Geometry: final body of the model. Coordinates: model frame, mm. Give positions to 0.01 mm unless a question says otherwise; leave off trailing zeros. Order: outer loops, then holes, each group sorted by start corner. A loop starts at its lowest first (then second) coordinate and runs counter-clockwise, first axis right, second up. Notation, with made-up numbers: (85.25, 7) - (140.25, 7) arc R35 cw to (140.25, 45) - close; hole circle Ø2 at (57.25, 52.5). An arc over 180 degrees is marked (long way). Use one line per item in the form item = value.
Autodesk Inventor part; units mm, degrees
ref_plane "YZ Plane" through (0, 0, 0) normal (1, 0, 0) x (0, 1, 0)
ref_plane "XZ Plane" through (0, 0, 0) normal (0, 1, 0) x (-1, 0, 0)
ref_plane "XY Plane" through (0, 0, 0) normal (0, 0, 1) x (1, 0, 0)
sketch "Sketch1" plane through (0, 0, 0) normal (0, 1, 0) x (-1, 0, 0)
  line L0 (11.02, 0) -> (0, 0)
  line L1 (-5, -122) -> (0, -122)
  line L2 (11.02, 0) -> (11.02, -122)
  line L3 (11.02, 0) -> (133.02, 0) construction
  line L4 (11.02, -122) -> (0, -122)
  line L5 (0, -126) -> (0, -122)
  line L6 (-5, -126) -> (-5, -122)
  line L7 (0, -126) -> (-5, -126)
  line L8 (-35, -122) -> (-30, -122)
  line L9 (-30, 0) -> (-35, 0)
  line L10 (0, -122) -> (-35, -122)
  line L11 (-35, -122) -> (-35, 0)
  line L12 (0, 0) -> (-35, 0)
  line L13 (-35, 0) -> (-35, 4)
  line L14 (-35, 4) -> (-30, 4)
  line L15 (-30, 0) -> (-30, 4)
  line L16 (-20, 0) -> (-20, 4)
  line L17 (-25, 4) -> (-20, 4)
  line L18 (-25, 0) -> (-25, 4)
  line L19 (-15, 0) -> (-15, 4)
  line L20 (-15, 4) -> (-10, 4)
  line L21 (-10, 0) -> (-10, 4)
  line L22 (0, 0) -> (0, 4)
  line L23 (-5, 4) -> (0, 4)
  line L24 (-5, 0) -> (-5, 4)
  line L25 (0, -126) -> (-5, -126)
  line L26 (-10, -126) -> (-10, -122)
  line L27 (-10, -126) -> (-15, -126)
  line L28 (-15, -126) -> (-15, -122)
  line L29 (-20, -126) -> (-20, -122)
  line L30 (-20, -126) -> (-25, -126)
  line L31 (-25, -126) -> (-25, -122)
  line L32 (-30, -126) -> (-30, -122)
  line L33 (-30, -126) -> (-35, -126)
  line L34 (-35, -126) -> (-35, -122)
  dimension "d0" = 90
extrude "Extrusion1" add sketch "Sketch1" along normal blind 4
properties part number "Angle_Zwischenebene"
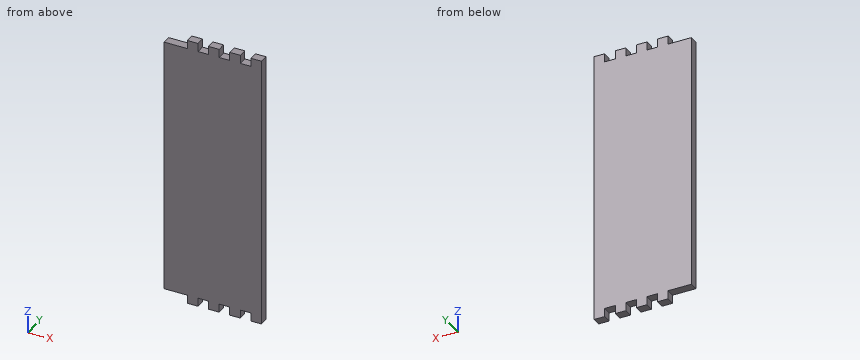
(1) Contact query for flat-ended pins moving along their axis: pin 1 Ø2 at (y, z) = (2.5, -124.5) entering from -X; pin 2 Ø1.2 at (x, y) = (16.5, 2.5) entering from -Z; pin 3 Ø1.2 at (x, y) = (18, 2) entering from +Z. Output: stop coordinate, or through.
Computed values:
pin_1 = 0
pin_2 = -122
pin_3 = 0
(2) Ray query, line 1 along Z through (x, y) = (7.5, 0.65). Return the intervals inside material, ascending.
Computed values:
line_1 = -122 to 0
(3) Cut plane B-B on x = 8. Output: boundary loops of the cut face in (y, z).
Computed values:
outline = (0, -122) - (4, -122) - (4, 0) - (0, 0) - close
